Drawing for the job (mm, zero at the part's lowest x, y, z). A direction names the side the tool comes from. Give positions to 0.01 mm unless a question says otherwise; leave off trailing zeros. Order: outer loops, then holes, each group sorted by start corner. A loop starts at its lowest first (then second) coordinate and runs counter-clockwise, first axis right, second up. Notation, with made-up numbers: M -18,-4.75 L -10,-4.75 A21 cw -10,21.25 Z; hole C 3.5,66.5 d10. An arc over 180 degrees is marked long. One line per item, written item: value.
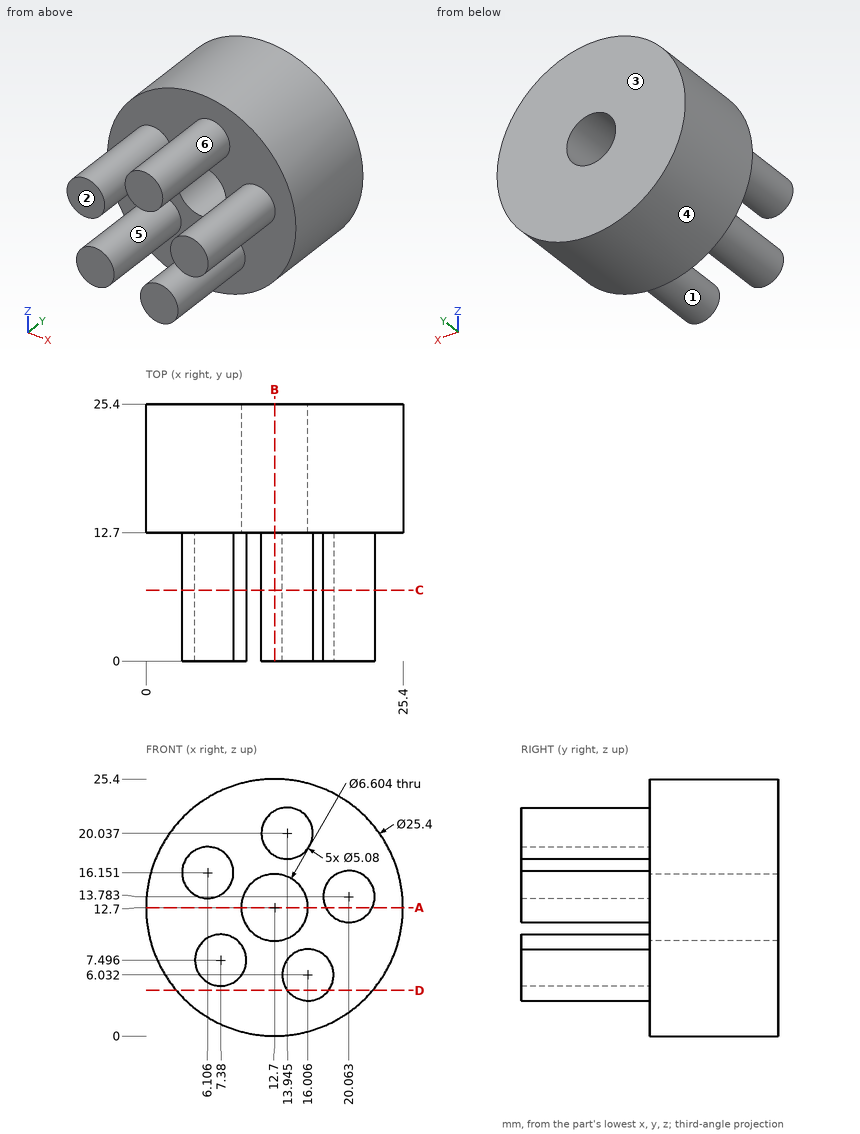
1) Saw through at A-A, the plane z = 12.7. Write the cut outline in (x, y) (1 decimal), then the cut area to 3 significant figures.
Check values:
outline: M 0,12.7 L 9.4,12.7 L 9.4,25.4 L 0,25.4 Z; M 16,12.7 L 17.8,12.7 L 17.8,0 L 22.4,0 L 22.4,12.7 L 25.4,12.7 L 25.4,25.4 L 16,25.4 Z
area: 297 mm^2
2) Saw through at D-D, the plane z = 4.5. Write the cut outline in (x, y), then the cut area to 3 significant figures.
Check values:
outline: M 3,12.7 L 13.98,12.7 L 13.98,0 L 18.03,0 L 18.03,12.7 L 22.4,12.7 L 22.4,25.4 L 3,25.4 Z
area: 298 mm^2
3) Saw through at B-B, the plane x = 12.7. Write the cut outline in (y, z), then the cut area to 3 significant figures.
Check values:
outline: M 0,17.82 L 12.7,17.82 L 12.7,16 L 25.4,16 L 25.4,25.4 L 12.7,25.4 L 12.7,22.25 L 0,22.25 Z; M 12.7,0 L 25.4,0 L 25.4,9.4 L 12.7,9.4 Z
area: 295 mm^2
4) Saw through at C-C, the plane y = 7. Write the cut outline in (x, z) (1 decimal), then the cut area to 3 significant figures.
Check values:
outline: C 6.1,16.2 d5.1; C 7.4,7.5 d5.1; C 13.9,20 d5.1; C 16,6 d5.1; C 20.1,13.8 d5.1
area: 101 mm^2
5) Pin check, flat tips, straight feed: pin 1 (12 mm diameter, centred on y = 11.5, z = 22.5, fed in from -X); pin 2 (8 mm diameter, centred on x = 22, y = 6.5, fed in from +Z); pin 3 (5 mm diameter, centred on x = 3, z = 11, fed in from -Y). Stop position of each tip, or through.
Check values:
pin 1: x = 0.62
pin 2: z = 16.32
pin 3: y = 12.7
6) Tool access for the marked faces 1 and 2: list every direction of +Z, -Z, +X, -X, +Y, -Y with a clear straight run to the whole face (end or side of a thin tool).
Check values:
face 1: -Y
face 2: +Z, -Z, +X, -X, -Y
7) Mould opens along Z. For the marked faces 3, 4, 5 and 6 say: released by +Z, released by -Z, zero draft, split by the parting line, or undercut.
Check values:
face 3: zero draft
face 4: split by the parting line
face 5: undercut
face 6: undercut
8) Drill centre lines: probe 1 along Y at (x, z) = (17.5, 11.75); probe 2 along Z at (x, y) = (5.5, 8) (1 decimal); probe 3 along X at (y, z) = (7.25, 20) (1 decimal). Where is each one in solid material? Low to high. Write a range as from..to.
Check values:
probe 1: 12.7..25.4
probe 2: 5.8..9.2, 13.7..18.6
probe 3: 11.4..16.5
